Can you work these out from the model? Positions are in its coordinate system, mm. Round coordinates to 2 decimals unless told otherwise and drop trailing zeros. Loops run counter-clockwise (first coordinate to the right, second up) from the corner with the lowest first, then second, coordinate; pieces in that order, holes last. Notation, with made-up numbers: (67.5, -27.5) - (85.5, -27.5) arc R22 ccw to (85.5, -5.5) - close; hole circle Ø3 at (-33.75, -39.5). An arc over 180 degrees is marked (long way). Answer as CSV lines item,"result".
```python
from build123d import *

# Parameters (mm, degrees)
SKETCH1_R           = 1
BOSS_EXTRUDE1_DEPTH = 2
MOVE_FACE1_BY       = 0.25


with BuildPart() as part:
    # Sketch1 → Boss-Extrude1 (new body)
    with BuildSketch(Plane(origin=(0, 0, 0), x_dir=(1, 0, 0), z_dir=(0, 1, 0))):
        with BuildLine():
            Line((-2.25, 0), (-2.25, 11.5))
            ThreePointArc((-2.25, 11.5), (0, 13.75), (2.25, 11.5))
            Line((2.25, 11.5), (2.25, 0))
            ThreePointArc((2.25, 0), (0, -2.25), (-2.25, 0))
        make_face()
        with Locations(Location((0, 5.75, 0), (0, 0, 270))):
            Circle(SKETCH1_R, mode=Mode.SUBTRACT)
    extrude(amount=BOSS_EXTRUDE1_DEPTH)

    # Move Face1: a curved face moved inward by 0.25
    add(Solid.thicken(part.faces().sort_by_distance((0, 1, -6.75))[0], -MOVE_FACE1_BY), mode=Mode.SUBTRACT)


solid = part.part
```
Q1. I'm going to push a flat-ended pin straight in: pin 1 Ø2 at (x, z) = (0, -5.75) entering from +Y. Where does the tip first touch, or does it pass through?
Checks:
pin 1,"through"
Q2. We'd pull the mould along X, two halves only. Please class faces 1 (the cylindrical face through (0, 1, -7)), 2 (the cylindrical face through (-0.05, 0.99, -13.75)), 3 (the flat face through (-2.25, 1, -6)): pulls with the +X half, pulls with the -X half, needs draft (parallel to the pull), parting line crosses it, or undercut.
Checks:
face 1,"undercut"
face 2,"parting line crosses it"
face 3,"pulls with the -X half"
Q3. Imagine slicing it at D-D (z = 0.5). Write out the boundary of the cut face in (x, y).
Checks:
outline,"(-2.19, 0) - (2.19, 0) - (2.19, 2) - (-2.19, 2) - close"
Q4. Imagine slicing it at A-A (z = -6.75). Write out the boundary of the cut face in (x, y).
Checks:
outline,"(-2.25, 0) - (-0.75, 0) - (-0.75, 2) - (-2.25, 2) - close; (0.75, 0) - (2.25, 0) - (2.25, 2) - (0.75, 2) - close"
Q5. Imagine slicing it at C-C (y = 1.2). Write out the boundary of the cut face in (x, z).
Checks:
outline,"(-2.25, -11.5) arc R2.25 ccw to (2.25, -11.5) - (2.25, 0) arc R2.25 ccw to (-2.25, 0) - close; hole circle Ø2.5 at (0, -5.75)"
Q6. If I drill on line 1 along X through (y, z) = (1.45, -5.75); line 2 along Z through (x, y) = (0.05, 1.55); line 3 along X through (y, z) = (1.3, -5), over which ranges is the centre line in solid material (lowest first)? Write a range as [from, to].
Checks:
line 1,"[-2.25, -1.25], [1.25, 2.25]"
line 2,"[-13.75, -7], [-4.5, 2.25]"
line 3,"[-2.25, -1], [1, 2.25]"
Q7. Imagine slicing it at B-B (x = 0). Write out the boundary of the cut face in (y, z), then the cut area to 3 significant figures.
Checks:
outline,"(0, -13.75) - (2, -13.75) - (2, -7) - (0, -7) - close; (0, -4.5) - (2, -4.5) - (2, 2.25) - (0, 2.25) - close"
area,"27.0 mm²"
